```python
from build123d import *

# Parameters (mm, degrees)
F0_R          = 12.7
F1_DEPTH      = 1.30175
F1_DEPTH_BACK = 1.30175
F2_R          = 12.573
F3_DEPTH      = 5.08
F4_R          = 12.573
F5_DEPTH      = 5.08


with BuildPart() as f1:
    # F0 (on Front) → F1 (new body, two sides)
    with BuildSketch(Plane.XZ) as f1_sk:
        Circle(F0_R)
    extrude(amount=F1_DEPTH)
    extrude(f1_sk.sketch, amount=-F1_DEPTH_BACK)

    # F2 (on face) → F3 (join)
    with BuildSketch(Plane.XZ.offset(1.30175)):
        Circle(F2_R)
    extrude(amount=F3_DEPTH)

    # F4 (on face) → F5 (join)
    with BuildSketch(Plane(origin=(0, 1.30175, 0), x_dir=(-1, 0, 0), z_dir=(0, 1, 0))):
        Circle(F4_R)
    extrude(amount=F5_DEPTH)


solid = f1.part
```
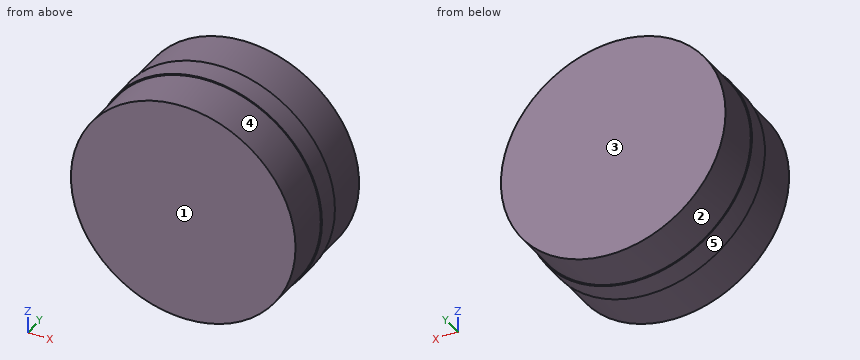
Geometry: final body of the model. Coordinates: model frame, mm. Face numbers are marked on the shaded views. A direction names the side the tool comes from. Round coordinates to 2 decimals unless told otherwise and drop trailing zeros. Order: outer loops, then holes, each group sorted by start corner. A loop starts at its lowest first (then second) coordinate and runs counter-clockwise, first axis right, second up. Notation, with made-up numbers: M 88.5,-26 L 136.5,-26 A31 cw 136.5,10 Z; hole C 79.5,6.5 d1. An arc over 180 degrees is marked long. Use one line per item in the form item = value. Start each with the question number.
Q1. Cut plane A-A (x = 3). Return loops of the section in (y, z).
Q2. Mould query, pull axis Y, two halves, no side actions, for the marked faces 1, 2 and 3. Classes: +Y half, -Y half, draft (parallel to the pull), parting line (faces both ways), or undercut.
Q3. Cut plane C-C (y = 2.5). Return loops of the section in (x, z).
Q4. Pin query (flat end, axial travel): pin 1 Ø6 at (y, z) = (4, 6) entering from +X; pin 2 Ø4 at (y, z) = (-4.5, 6.5) entering from -X. Return the tip coordinate at first contact, or that it passes through.
Q5. Cut plane D-D (y = 0.75). Return loops of the section in (x, z).
Q6. Cut plane B-B (z = 7.75). Return loops of the section in (x, y).
Q7. Access query for the marked faces 4 and 5. Directions: +Z, -Z, +X, -X, +Y, -Y. A direction counts if a zero-diameter tool reaches every point of the face in a straight line with its end or side. Return the directions, or none.
Q8. Material intervals for line 1 (Z direction, x = 0.25, y = 0); line 2 (X direction, y = 0.5, z = -1.75); line 3 (Y direction, x = -7.75, z = 10), sorted ascending. Write a range as [from, to].
Geometry results:
q1.outline = M -6.38,-12.21 L -1.3,-12.21 L -1.3,-12.34 L 1.3,-12.34 L 1.3,-12.21 L 6.38,-12.21 L 6.38,12.21 L 1.3,12.21 L 1.3,12.34 L -1.3,12.34 L -1.3,12.21 L -6.38,12.21 Z
q2.face_1 = -Y half
q2.face_2 = draft
q2.face_3 = +Y half
q3.outline = C 0,0 d25.15
q4.pin_1 = 12.21
q4.pin_2 = -11.74
q5.outline = C 0,0 d25.4
q6.outline = M -10.06,-1.3 L -9.9,-1.3 L -9.9,-6.38 L 9.9,-6.38 L 9.9,-1.3 L 10.06,-1.3 L 10.06,1.3 L 9.9,1.3 L 9.9,6.38 L -9.9,6.38 L -9.9,1.3 L -10.06,1.3 Z
q7.face_4 = -Y
q7.face_5 = +Y, -Y
q8.line_1 = [-12.7, 12.7]
q8.line_2 = [-12.58, 12.58]
q8.line_3 = [-1.3, 1.3]
